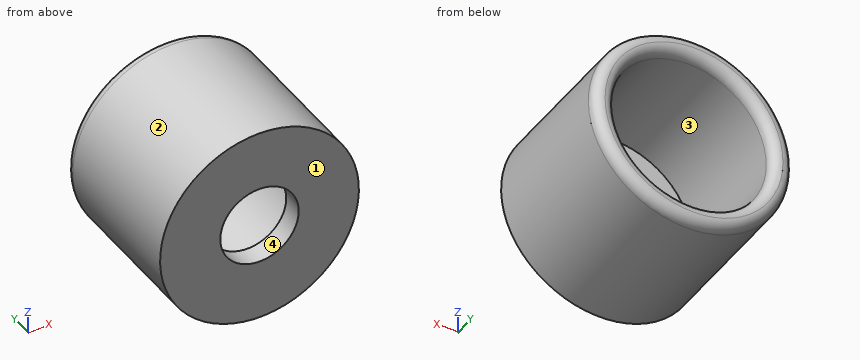
```python
from build123d import *

# Parameters (mm, degrees)
SKETCH_1_R      = 3.8
SKETCH_1_R_2    = 3
EXTRUDE_1_DEPTH = 6
SKETCH_1_13_R   = 3
SKETCH_1_13_R_2 = 1.5
EXTRUDE_2_DEPTH = 0.8
FILLET_1_R      = 0.4


with BuildPart() as part:
    # 草图1 → 凸台-拉伸1 (new body)
    with BuildSketch(Plane(origin=(0, 0, 0), x_dir=(1, 0, 0), z_dir=(0, 1, 0))):
        with Locations(Location((-1.835e-06, 48.853027267, 0), (0, 0, 270))):
            Circle(SKETCH_1_R)
        with Locations(Location((-1.835e-06, 48.853027267, 0), (0, 0, 270))):
            Circle(SKETCH_1_R_2, mode=Mode.SUBTRACT)
    extrude(amount=EXTRUDE_1_DEPTH)

    # 草图1<13> → 凸台-拉伸2 (add)
    with BuildSketch(Plane(origin=(0, 0, 0), x_dir=(1, 0, 0), z_dir=(0, 1, 0))):
        with Locations(Location((-1.835e-06, 48.853027267, 0), (0, 0, 270))):
            Circle(SKETCH_1_13_R)
        with Locations(Location((-1.835e-06, 48.853027267, 0), (0, 0, 270))):
            Circle(SKETCH_1_13_R_2, mode=Mode.SUBTRACT)
    extrude(amount=EXTRUDE_2_DEPTH)

    # 圆角1
    fillet_1_edges = [part.edges().sort_by_distance(p)[0] for p in [
        (-1.835e-06, 6, -52.653027267),
        (-1.835e-06, 6, -51.853027267),
    ]]
    fillet(fillet_1_edges, radius=FILLET_1_R - 0.0001)  # a hair under: the kernel refuses the full size


solid = part.part
```
Part model, mm, in its own coordinate system. Face numbers are marked on the shaded views. Coordinates: 2 decimals unless noted, no trailing zeros. Write each loop counter-clockwise with the first axis right and the second up, starting at its lowest first coordinate (ties: lowest second). Pieces come first, ordered by that corner, then holes.
Item 1: Pin check, flat tips, straight feed: pin 1 (2 mm diameter, centred on y = 3, z = -49.5, fed in from +X); pin 2 (1.5 mm diameter, centred on x = 1.5, y = 3, fed in from +Z). Stop position of each tip, or through.
Item 2: Probe line 1 (Y direction, x = -2.25, z = -50.25); line 2 (Z direction, x = 2.5, y = 4.5); line 3 (Z direction, x = 2, y = 3). List the from-to ranges inside material, lowest first.
Item 3: Slice it at A-A (y = 2.5). Write the cut outline in (x, z), and give its area (3 significant figures).
Item 4: Mould opens along Z. For the marked faces 1, 2, 3 and 4 say: released by +Z, released by -Z, zero draft, split by the parting line, or undercut.
Results found:
1. pin 1: stops at x = 3.8
1. pin 2: stops at z = -45.13
2. line 1: y = 0 to 0.8
2. line 2: z = -51.71 to -50.51, -47.19 to -45.99
2. line 3: z = -52.08 to -51.09, -46.62 to -45.62
3. outline: circle Ø7.6 at (0, -48.85); hole circle Ø6 at (0, -48.85)
3. area: 17.1 mm2
4. face 1: zero draft
4. face 2: split by the parting line
4. face 3: undercut
4. face 4: undercut
